```python
from build123d import *

# Parameters (mm, degrees)
SKETCH1_W           = 3
SKETCH1_H           = 110
EXTRUDE_THIN1_DEPTH = 90
CAVITY1_START       = 14.397705985
CAVITY1_OUTLINE_W   = 3
CAVITY1_OUTLINE_H   = 3
CAVITY1_DEPTH       = 30
CAVITY1_START_2     = -25.602294015
CAVITY1_2_OUTLINE_W = 3
CAVITY1_2_OUTLINE_H = 3
CAVITY1_2_DEPTH     = 20
CAVITY1_START_3     = 64.397705985
CAVITY1_3_OUTLINE_W = 3
CAVITY1_3_OUTLINE_H = 3
CAVITY1_3_DEPTH     = 20
FILLET1_R           = 2


# Read off the part's stored shape, not the designer's step: Cavity1
with BuildPart() as part:
    # Sketch1 → Extrude-Thin1 (new body)
    with BuildSketch(Plane.XY.offset(1.5)):
        with Locations((-5.414893617, 29.397705985)):
            Rectangle(SKETCH1_W, SKETCH1_H)
    extrude(amount=-EXTRUDE_THIN1_DEPTH)

    # Cavity1 outline → Cavity1 (cut)
    with BuildSketch(Plane(origin=(0, 0, 0), x_dir=(1, 0, 0), z_dir=(0, 1, 0)).offset(CAVITY1_START)):
        with Locations((-5.414893617, 87)):
            Rectangle(CAVITY1_OUTLINE_W, CAVITY1_OUTLINE_H)
        with Locations((-5.414893617, 0)):
            Rectangle(CAVITY1_OUTLINE_W, CAVITY1_OUTLINE_H)
    extrude(amount=CAVITY1_DEPTH, mode=Mode.SUBTRACT)

    # Cavity1 2 outline → Cavity1 2 (cut)
    with BuildSketch(Plane(origin=(0, 0, 0), x_dir=(1, 0, 0), z_dir=(0, 1, 0)).offset(CAVITY1_START_2)):
        with Locations((-5.414893617, 87)):
            Rectangle(CAVITY1_2_OUTLINE_W, CAVITY1_2_OUTLINE_H)
        with Locations((-5.414893617, 0)):
            Rectangle(CAVITY1_2_OUTLINE_W, CAVITY1_2_OUTLINE_H)
    extrude(amount=CAVITY1_2_DEPTH, mode=Mode.SUBTRACT)

    # Cavity1 3 outline → Cavity1 3 (cut)
    with BuildSketch(Plane(origin=(0, 0, 0), x_dir=(1, 0, 0), z_dir=(0, 1, 0)).offset(CAVITY1_START_3)):
        with Locations((-5.414893617, 87)):
            Rectangle(CAVITY1_3_OUTLINE_W, CAVITY1_3_OUTLINE_H)
        with Locations((-5.414893617, 0)):
            Rectangle(CAVITY1_3_OUTLINE_W, CAVITY1_3_OUTLINE_H)
    extrude(amount=CAVITY1_3_DEPTH, mode=Mode.SUBTRACT)

    # Fillet1
    fillet1_edges = [part.edges().sort_by_distance(p)[0] for p in [
        (-5.414893617, -25.602294015, -85.5),
        (-5.414893617, 84.397705985, -85.5),
        (-5.414893617, -25.602294015, -1.5),
        (-5.414893617, 84.397705985, -1.5),
    ]]
    fillet(fillet1_edges, radius=FILLET1_R)


solid = part.part
```
Input: part model. Units: mm. Frame: model coordinates. A direction names the side the tool comes from. Coordinates: 2 decimals unless noted, no trailing zeros. Write each loop counter-clockwise with the first axis right and the second up, starting at its lowest first coordinate (ties: lowest second). Pieces come first, ordered by that corner, then holes.
1) Mould query, pull axis Y, two halves, no side actions, for faces 1 (the flat face through (-5, -5.602, -87)), 2 (the flat face through (-5, 5, -88.5)), 3 (the flat face through (-5, 14.398, 0)). Classes: pulls with the +Y half, pulls with the -Y half, needs draft (parallel to the pull), parting line crosses it, or undercut.
2) Pin query (flat end, axial travel): pin 1 Ø1.5 at (x, y) = (-6, 71) entering from -Z; pin 2 Ø1.5 at (x, z) = (-6, 0) entering from -Y; pin 3 Ø1.5 at (x, z) = (-6, 0) entering from +Y. Return the tip coordinate at first contact, or that it passes through.
3) Section B-B on y = 27.5. Output: boundary loops of the cut face in (x, z), and give its area (3 significant figures).
4) Material intervals for line 1 along Z through (x, y) = (-6.2, -18.5), sorted ascending.
5) Section A-A on x = -5.7. Output: boundary loops of the cut face in (y, z), and give its area (3 significant figures).
6) Set-up query: faces 4 (the flat face through (-5, 29, -1.5)), 5 (the flat face through (-5, 64.398, 0)), 6 (the flat face through (-5, 64.398, -87)), 7 (the flat face through (-5, 14.398, -87)), 8 (the flat face through (-5, -15, -1.5)). Return all of +Z, -Z, +X, -X, +Y, -Y with unobstructed straight access to the full face (end or side cutting, diameter ignored); none if empty.
Check result:
1. face 1: pulls with the -Y half
1. face 2: needs draft
1. face 3: undercut
2. pin 1: stops at z = -85.5
2. pin 2: stops at y = -5.6
2. pin 3: stops at y = 64.4
3. outline: (-6.91, -85.5) - (-3.91, -85.5) - (-3.91, -1.5) - (-6.91, -1.5) - close
3. area: 252 mm2
4. line 1: z = -85.5 to -1.5
5. outline: (-25.6, -83.5) arc R2 ccw to (-23.6, -85.5) - (-5.6, -85.5) - (-5.6, -88.5) - (14.4, -88.5) - (14.4, -85.5) - (44.4, -85.5) - (44.4, -88.5) - (64.4, -88.5) - (64.4, -85.5) - (82.4, -85.5) arc R2 ccw to (84.4, -83.5) - (84.4, -3.5) arc R2 ccw to (82.4, -1.5) - (64.4, -1.5) - (64.4, 1.5) - (44.4, 1.5) - (44.4, -1.5) - (14.4, -1.5) - (14.4, 1.5) - (-5.6, 1.5) - (-5.6, -1.5) - (-23.6, -1.5) arc R2 ccw to (-25.6, -3.5) - close
5. area: 9,480 mm2
6. face 4: +Z, +X, -X
6. face 5: +Z, +X, -X, +Y
6. face 6: -Z, +X, -X, +Y
6. face 7: -Z, +X, -X
6. face 8: +Z, +X, -X, -Y
